Input: part model. Units: mm. Frame: model coordinates. A direction names the side the tool comes from. Give positions to 0.01 mm unless a question says otherwise; leave off trailing zeros. Write each loop counter-clockwise with the first axis right and the second up, starting at its lowest first coordinate (ties: lowest second). Pieces come first, ordered by that corner, then holes. Notation, with made-up numbers: M 89,-24.5 L 142,-24.5 A13 cw 142,-4.5 Z; hole C -39,52.5 d7. An arc over 180 degrees is marked long. Use CSV: the item, a comma, the result in double quotes. Start each with the question number.
from build123d import *

# Parameters (mm, degrees)
SKETCH5_R           = 3.175
BOSS_EXTRUDE3_DEPTH = 95.25
BOSS_EXTRUDE4_DEPTH = 3.96875
SKETCH8_OUTSIDE_W   = 380.412
SKETCH8_OUTSIDE_H   = 382.132
SKETCH8_OUTSIDE_R   = 5.55625
CUT_EXTRUDE3_DEPTH  = 100.21875
CUT_EXTRUDE3_TAPER  = 60
CUT_EXTRUDE4_DEPTH  = 0.254
CIRPATTERN1_COUNT   = 3


with BuildPart() as part:
    # Sketch5 → Boss-Extrude3 (new body)
    with BuildSketch(Plane(origin=(49.609375, 0, 0), x_dir=(0, 0, -1), z_dir=(1, 0, 0))):
        Circle(SKETCH5_R)
    extrude(amount=-BOSS_EXTRUDE3_DEPTH)

    # Sketch11 → Revolve1 (revolve)
    with BuildSketch(Plane.XY):
        Polygon((-45.640625, 3.175), (-45.640625, 0), (33.734375, 0), (30.559375, 3.175), align=None)
    revolve(axis=Axis((-45.640625, 0, 0), (1, 0, 0)))

    # Sketch6 → Boss-Extrude4 (add)
    with BuildSketch(Plane.ZY.offset(45.640625)):
        Polygon((5.55625, 3.207902433), (0, 6.415804866), (-5.55625, 3.207902433), (-5.55625, -3.207902433), (0, -6.415804866), (5.55625, -3.207902433), align=None)
    extrude(amount=BOSS_EXTRUDE4_DEPTH)

    # Sketch8 outside → Cut-Extrude3 (cut, through all)
    with BuildSketch(Plane.ZY.offset(49.609375)):
        Rectangle(SKETCH8_OUTSIDE_W, SKETCH8_OUTSIDE_H)
        Circle(SKETCH8_OUTSIDE_R, mode=Mode.SUBTRACT)
    extrude(amount=-CUT_EXTRUDE3_DEPTH, taper=CUT_EXTRUDE3_TAPER, mode=Mode.SUBTRACT)

    # Sketch12 → Cut-Extrude4 (cut)
    with BuildSketch(Plane.ZY.offset(49.609375)):
        with BuildLine():
            Line((0.1666875, 4.2783125), (0.1666875, 2.3891875))
            ThreePointArc((0.1666875, 2.3891875), (0, 2.2225), (-0.1666875, 2.3891875))
            Line((-0.1666875, 2.3891875), (-0.1666875, 4.2783125))
            ThreePointArc((-0.1666875, 4.2783125), (0, 4.445), (0.1666875, 4.2783125))
        make_face()
    cut_extrude4 = extrude(amount=-CUT_EXTRUDE4_DEPTH, mode=Mode.SUBTRACT)

    # CirPattern1: Cut-Extrude4 ×3 about axis
    cirpattern1_axis = Axis((0, 0, 0), (1, 0, 0))
    for i in range(1, CIRPATTERN1_COUNT):
        add(cut_extrude4.rotate(cirpattern1_axis, i * 360 / CIRPATTERN1_COUNT), mode=Mode.SUBTRACT)


solid = part.part
Q1. Set-up query: faces 1 (the flat face through (-47.597, 4.834, -2.739)), 2 (the flat face through (-45.641, -3, -3)). Return all of +Z, -Z, +X, -X, +Y, -Y with unobstructed straight access to the full face (end or side cutting, diameter ignored); none if empty.
Q2. First-contact query: pin 1 Ø3 at (x, y) = (0.5, -0.5) entering from +Z (3 decimals); pin 2 Ø5 at (x, y) = (-39.5, -3.5) entering from +Z; pin 3 Ø6 at (x, z) = (-32, 3) entering from -Y (3 decimals). Flat tips, straight axial feed; report the tip coordinate or a pass-through.
Q3. Section A-A, the plane x = 22.5. Return the cut outline in (y, z) (3 decimals), and give its area (3 significant figures).
Q4. Material intervals for L1, parallel to X at y = -1.5, z = 2.5; L2, parallel to X at y = -2.5, z = 5; L3, parallel to Z at x = 39, y = 0 (3 decimals), sorted ascending. Write a range as [from, to].
Check result:
1,face 1,"-Z, +X, -X, +Y"
1,face 2,"+X"
2,pin 1,"stops at z = 3.175"
2,pin 2,"stops at z = 3.01"
2,pin 3,"stops at y = -3.175"
3,outline,"C 0,0 d6.35"
3,area,"31.7 mm²"
4,L1,"x = [-49.36, 49.61]"
4,L2,"x = [-49.59, -45.64]"
4,L3,"z = [-3.175, 3.175]"
